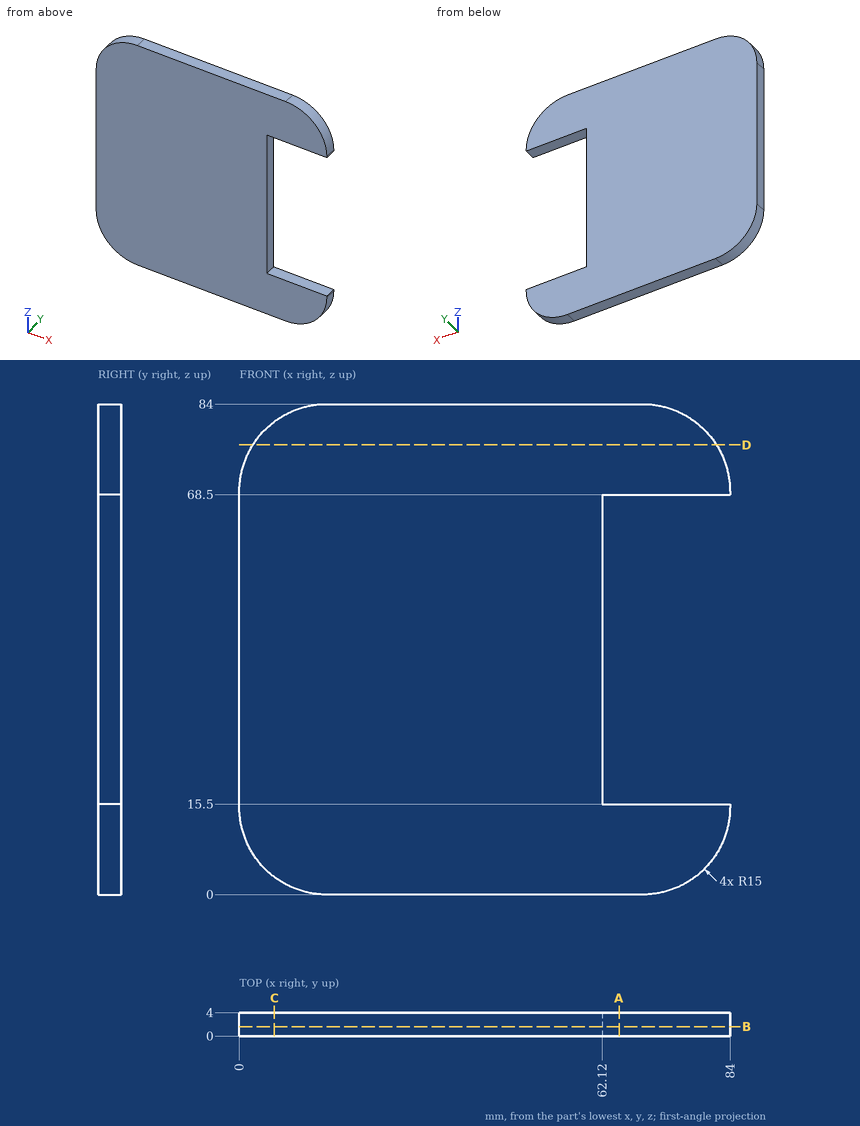
The figure shows three views and two pictorial views of one solid part (mm, origin at its lowest corner). Answer the questions. Round coordinates to 2 decimals unless told otherwise and drop trailing zeros. Write each loop counter-clockwise with the first axis right and the second up, starting at its lowest first coordinate (ties: lowest second). Pieces come first, ordered by that corner, then holes. Notation, with made-up numbers: M 80.25,9 L 121.25,9 A10 cw 121.25,18 Z; hole C -14.75,2 d5. An arc over 180 degrees is marked long. Use a Markdown table: item, result.
1) The part is cut by section C-C on x = 6. Give the vertices of the cut face in (y, z), plus the area to 3 significant figures.
Taken from the geometry:
| item | result |
|---|---|
| outline | M 0,3 L 4,3 L 4,81 L 0,81 Z |
| area | 312 mm2 |
2) Consider line 1 (Z direction, x = 63, y = 0.95); line 2 (X direction, y = 1.8, z = 57); line 3 (Z direction, x = 80.5, y = 0.65). Determine where each line is inside the solid, lowest interval first. Write a range as [from, to].
Taken from the geometry:
| item | result |
|---|---|
| line 1 | z = [0, 15.5], [68.5, 84] |
| line 2 | x = [0, 62.12] |
| line 3 | z = [5.37, 15.5], [68.5, 78.63] |
3) The part is cut by section B-B on y = 1.6. Give the vertices of the cut face in (x, z), plus the area to 3 significant figures.
Taken from the geometry:
| item | result |
|---|---|
| outline | M 0,15 A15 ccw 15,0 L 69,0 A15 ccw 84,15 L 84,15.5 L 62.12,15.5 L 62.12,68.5 L 84,68.5 L 84,69 A15 ccw 69,84 L 15,84 A15 ccw 0,69 Z |
| area | 5,700 mm2 |
4) The part is cut by section A-A on x = 65. Give the vertices of the cut face in (y, z), plus the area to 3 significant figures.
Taken from the geometry:
| item | result |
|---|---|
| outline | M 0,0 L 4,0 L 4,15.5 L 0,15.5 Z; M 0,68.5 L 4,68.5 L 4,84 L 0,84 Z |
| area | 124 mm2 |
5) The part is cut by section D-D on z = 77. Give the vertices of the cut face in (x, y), plus the area to 3 significant figures.
Taken from the geometry:
| item | result |
|---|---|
| outline | M 2.31,0 L 81.69,0 L 81.69,4 L 2.31,4 Z |
| area | 318 mm2 |
